Source: CAD feature listing. Evaluate the final solid. Frame: model axes, mm. Face numbers are marked on the shaded views. A direction names the side the tool comes from. Coordinates: 2 decimals unless noted, no trailing zeros. Write each loop counter-clockwise with the first axis right and the second up, starting at its lowest first coordinate (ties: lowest second). Pieces come first, ordered by that corner, then holes. Notation, with made-up numbers: (65.25, 1.5) - (86.25, 1.5) arc R3 ccw to (86.25, 6.5) - close; hole circle Ø7 at (59, 67). An arc over 180 degrees is marked (long way). One line per question, with ' | ' between items. Start each with the question number.
Q1. Cut plane C-C, the plane z = -1.75. Return loops of the section in (x, y).
Q2. Access query for the marked faces 1, 2, 3 and 4. Directions: +Z, -Z, +X, -X, +Y, -Y. A direction counts if a zero-diameter tool reaches every point of the face in a straight line with its end or side. Return the directions, or none.
Q3. Draft query along X for the marked faces 5, 6 and 7. Return one class per face: +X half, -X half, draft (parallel to the pull), parting line (faces both ways), or undercut.
Q4. Cut plane D-D, the plane z = -5.5. Return loops of the section in (x, y), plus the area to 3 significant figures.
Q5. Contact query for flat-ended pins moving along their axis: P1, Ø6, axis at x = 9, y = 4, coming from the -Z side; P2, Ø8, axis at y = 5.5, z = -7.5, coming from the -X side; P3, Ø3, axis at y = 8, z = 1.5, coming from the +X side; P4, Ø5, axis at x = 5.5, z = -8, coming from the -Y side. Output: stop coordinate, or through.
Q6. Cut plane A-A, the plane y = 0. Return loops of the section in (x, z).
Q7. Line query: line 1 (Y direction, x = 0, z = -4.75); line 2 (Z direction, x = 0, y = -6.45); line 3 (Y direction, x = 0, z = 4.5). Output: solid intervals per line, ascending.
Q8. Cut plane B-B, the plane x = 0. Return loops of the section in (y, z).
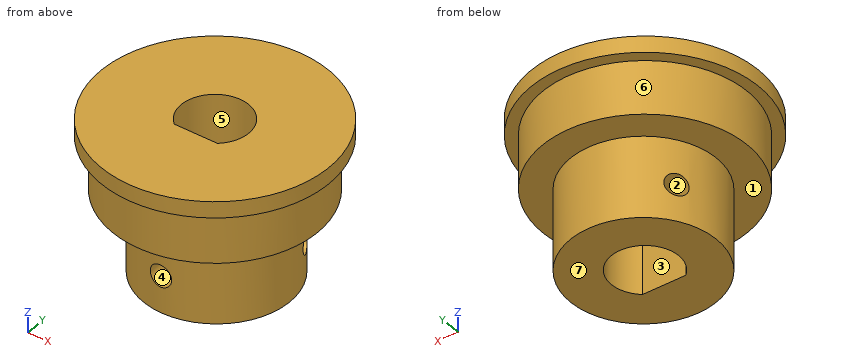
```python
from build123d import *

# Parameters (mm, degrees)
SKETCH_1_R               = 12.6
EXTRUDE_1_DEPTH          = 6.6
SKETCH_2_R               = 14
EXTRUDE_2_DEPTH          = 2
SKETCH_4_R               = 9
EXTRUDE_3_DEPTH          = 10
CUT_EXTRUDE_START        = -4
SKETCH_5_R               = 1.35
CUT_EXTRUDE_2_DEPTH      = 8
CUT_EXTRUDE_1_DEPTH      = 28.165419263
PATTERN_CIRCULAR_1_COUNT = 3


with BuildPart() as part:
    # 草图1 → 凸台-拉伸1 (new body)
    with BuildSketch(Plane.XY):
        Circle(SKETCH_1_R)
    extrude(amount=EXTRUDE_1_DEPTH)

    # 草图2 → 凸台-拉伸2 (add)
    with BuildSketch(Plane.XY.offset(6.6)):
        Circle(SKETCH_2_R)
    extrude(amount=EXTRUDE_2_DEPTH)

    # 草图4 → 凸台-拉伸3 (add)
    with BuildSketch(Plane(origin=(0, 0, 0), x_dir=(-1, 0, 0), z_dir=(0, 0, -1))):
        with Locations((-0.193153064, 0)):
            Circle(SKETCH_4_R)
    extrude(amount=EXTRUDE_3_DEPTH)

    # 草图5 → 切除-拉伸2 (cut)
    with BuildSketch(Plane(origin=(0, 0, 0), x_dir=(1, 0, 0), z_dir=(0, 1, 0)).offset(CUT_EXTRUDE_START)):
        with Locations(Location((0, 5.5, 0), (0, 0, 270))):
            Circle(SKETCH_5_R)
    cut_extrude_2 = extrude(amount=-CUT_EXTRUDE_2_DEPTH, mode=Mode.SUBTRACT)

    # 草图3 → 切除-拉伸1 (cut, through all)
    with BuildSketch(Plane.XY.offset(8.6)):
        with BuildLine():
            Line((-2.701851217, -3.15), (2.701851217, -3.15))
            ThreePointArc((2.701851217, -3.15), (0, 4.15), (-2.701851217, -3.15))
        make_face()
    extrude(amount=-CUT_EXTRUDE_1_DEPTH, mode=Mode.SUBTRACT)

    # 阵列(圆周)1: 切除-拉伸2 ×3 about axis
    pattern_circular_1_axis = Axis((0.193153064, 0, 0), (0, 0, 1))
    for i in range(1, PATTERN_CIRCULAR_1_COUNT):
        add(cut_extrude_2.rotate(pattern_circular_1_axis, i * 360 / PATTERN_CIRCULAR_1_COUNT), mode=Mode.SUBTRACT)


solid = part.part
```
Reply:
1) outline: circle Ø18 at (0.19, 0); hole (-2.7, -3.15) - (2.7, -3.15) arc R4.15 ccw (long way) to start
2) face 1: -Z | face 2: none | face 3: +Z, -Z | face 4: -Y
3) face 5: undercut | face 6: parting line | face 7: draft
4) outline: (-8.11, 3.46) arc R9 ccw to (-1.35, -8.87) - (-1.35, -4) - (1.35, -4) - (1.35, -8.93) arc R9 ccw to (8.64, 3.1) - (4.43, 0.66) - (3.08, 3) - (7.34, 5.46) arc R9 ccw to (-6.71, 5.77) - (-2.5, 3.34) - (-2.52, 3.29) arc R4.15 cw to (2.7, -3.15) - (-2.7, -3.15) arc R4.15 cw to (-4, 1.09) - close | area: 164 mm^2
5) P1: stops at z = -10 | P2: stops at x = -8.68 | P3: stops at x = 10.79 | P4: stops at y = -8.55
6) outline: (-14, 6.6) - (-12.6, 6.6) - (-12.6, 0) - (-8.81, 0) - (-8.81, -10) - (-4.15, -10) - (-4.15, 8.6) - (-14, 8.6) - close; (4.15, -10) - (9.19, -10) - (9.19, 0) - (12.6, 0) - (12.6, 6.6) - (14, 6.6) - (14, 8.6) - (4.15, 8.6) - close
7) line 1: y = -4 to -3.15, 4.15 to 9 | line 2: z = -10 to -6.85, -4.15 to 8.6 | line 3: y = -12.6 to -3.15, 4.15 to 12.6
8) outline: (-14, 6.6) - (-12.6, 6.6) - (-12.6, 0) - (-9, 0) - (-9, -4.15) - (-4, -4.15) - (-4, -6.85) - (-9, -6.85) - (-9, -10) - (-3.15, -10) - (-3.15, 8.6) - (-14, 8.6) - close; (4.15, -10) - (9, -10) - (9, 0) - (12.6, 0) - (12.6, 6.6) - (14, 6.6) - (14, 8.6) - (4.15, 8.6) - close
